Job drawing, mm, ordinate dimensions from the low corner. One solid piece. A direction names the side the tool comes from. Coordinates: 2 decimals unless noted, no trailing zeros. Order: outer loops, then holes, each group sorted by start corner. A loop starts at its lowest first (then second) coordinate and runs counter-clockwise, first axis right, second up. Notation, with made-up numbers: (66.25, -11) -> (110.25, -11) arc R26 ccw to (110.25, 24) -> close; hole circle Ø3 at (-8, -28). An arc over 180 degrees is marked (long way). Use CSV: the item, a comma, the result in double quotes. Start each with the question number.
(1) Cut at B-B on x = 9.4. Write the cut outline in (y, z).
(2) Tool access for the marked faces 1 and 2: list every direction of +Z, -Z, +X, -X, +Y, -Y with a clear straight run to the whole face (end or side of a thin tool).
(3) Cut at D-D on z = 12.5. Write the cut outline in (x, y) (1 decimal).
(4) Pin check, flat tips, straight feed: pin 1 Ø5 at (x, z) = (35, 33.84) entering from +Y; pin 2 Ø3 at (x, y) = (19, 1) entering from -Z. Stop position of each tip, or through.
(5) Cut at A-A on z = 31. Write the cut outline in (x, y).
(6) Probe L1, parallel to X at y = 19.5, z = 23; L2, parallel to Y at x = 8.5, z = 39; L3, parallel to Y at x = 1.55, z = 12.5 (1 decimal). List the from-to ranges inside material, lowest first.
(7) Cut at C-C on y = 37. Write the cut outline in (x, z).
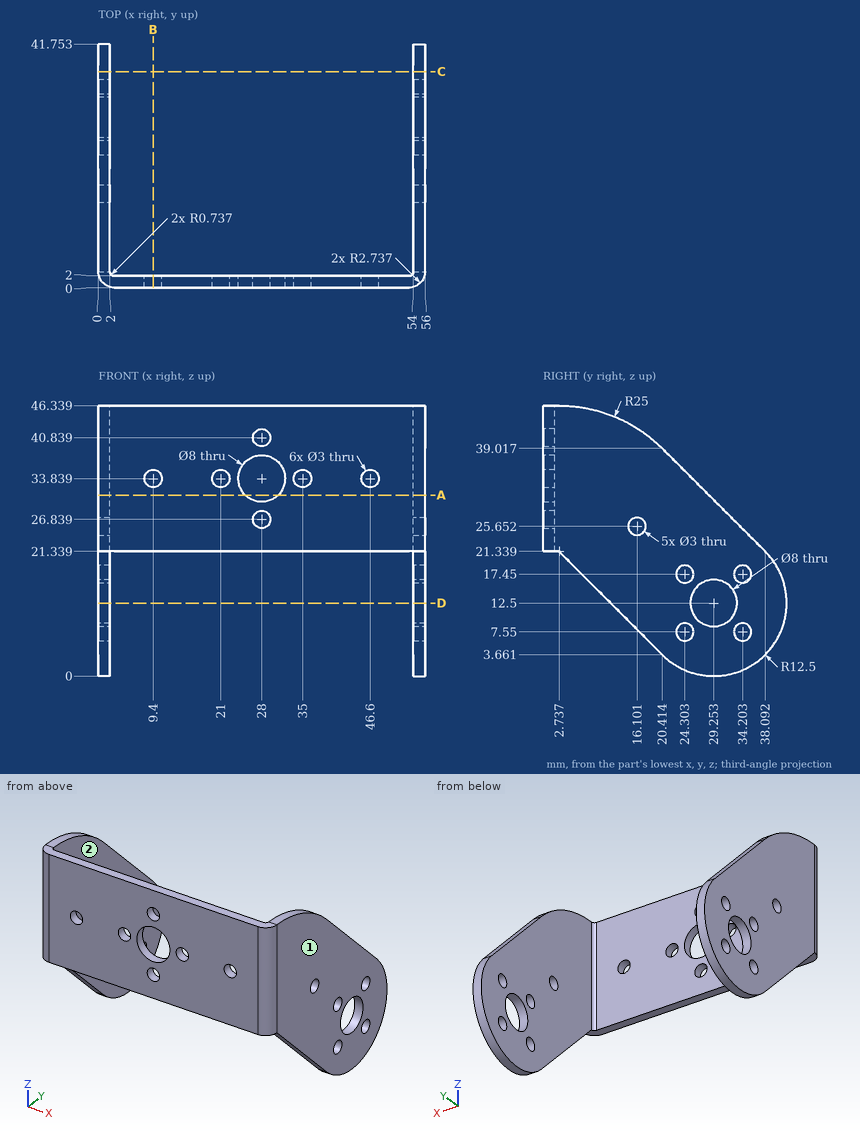
Outcome:
1,outline,"(0, 21.34) -> (2, 21.34) -> (2, 32.34) -> (0, 32.34) -> close; (0, 35.34) -> (2, 35.34) -> (2, 46.34) -> (0, 46.34) -> close"
2,face 1,"+Z, -Z, +X, +Y, -Y"
2,face 2,"+Z, -Z, +Y"
3,outline,"(0, 11.6) -> (2, 11.6) -> (2, 25.3) -> (0, 25.3) -> close; (0, 33.3) -> (2, 33.3) -> (2, 41.8) -> (0, 41.8) -> close; (54, 11.6) -> (56, 11.6) -> (56, 25.3) -> (54, 25.3) -> close; (54, 33.3) -> (56, 33.3) -> (56, 41.8) -> (54, 41.8) -> close"
4,pin 1,"y = 2"
4,pin 2,"z = 21.34"
5,outline,"(0, 2.74) arc R2.74 ccw to (2.74, 0) -> (25.18, 0) -> (25.18, 2) -> (2.74, 2) arc R0.74 cw to (2, 2.74) -> (2, 28.43) -> (0, 28.43) -> close; (30.82, 0) -> (53.26, 0) arc R2.74 ccw to (56, 2.74) -> (56, 28.43) -> (54, 28.43) -> (54, 2.74) arc R0.74 cw to (53.26, 2) -> (30.82, 2) -> close"
6,L1,"0 to 2, 54 to 56"
6,L2,"0 to 2"
6,L3,"11.6 to 25.3, 33.3 to 41.8"
7,outline,"(0, 2.69) -> (2, 2.69) -> (2, 22.43) -> (0, 22.43) -> close; (54, 2.69) -> (56, 2.69) -> (56, 22.43) -> (54, 22.43) -> close"
